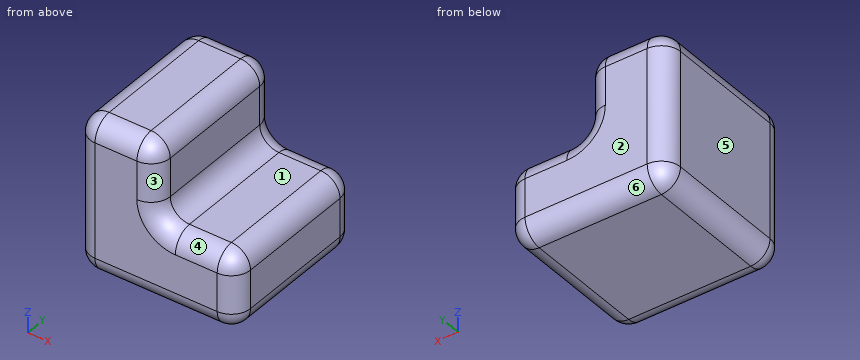
```python
from build123d import *

# Parameters (mm, degrees)
F0_W     = 83.6216490716
F0_H     = 83.1985995173
F1_DEPTH = 40
F2_W     = 41.8108245358
F2_H     = 83.1985995173
F3_DEPTH = 40
F4_F1_R  = 10
F4_F2_R  = 10


with BuildPart() as f1:
    # F0 (on Top) → F1 (new body)
    with BuildSketch(Plane.XY):
        with Locations((-17.3164242879, -4.335001111)):
            Rectangle(F0_W, F0_H)
    extrude(amount=F1_DEPTH)

    # F2 (on face) → F3 (join)
    with BuildSketch(Plane.XY.offset(40)):
        with Locations((-38.2218365557, -4.335001111)):
            Rectangle(F2_W, F2_H)
    extrude(amount=F3_DEPTH)

    # F4: fillet of radius 10 on 16 edges, made by hand

    # F4_f1
    f4_f1_edges = [f1.edges().sort_by_distance(p)[0] for p in [
        (-17.3164242879, -4.335001111, 40),
    ]]
    fillet(f4_f1_edges, radius=F4_F1_R)

    # F4_f2
    f4_f2_edges = [f1.edges().sort_by_distance(p)[0] for p in [
        (-17.3164242879, -4.335001111, 80),
        (-38.2218365557, -45.9343008697, 80),
        (-17.3164242879, -45.9343008697, 65),
        (-59.1272488236, -4.335001111, 80),
        (-38.2218365557, 37.2642986476, 80),
        (8.58898798, 37.2642986476, 40),
        (24.4944002479, -4.335001111, 40),
        (24.4944002479, -45.9343008697, 20),
        (24.4944002479, 37.2642986476, 20),
        (-17.3164242879, -45.9343008697, 0),
        (-59.1272488236, -45.9343008697, 40),
        (-59.1272488236, 37.2642986476, 40),
        (-59.1272488236, -4.335001111, 0),
        (-17.3164242879, 37.2642986476, 0),
        (24.4944002479, -4.335001111, 0),
        (-14.3874920997, 37.2642986476, 42.9289321881),
        (-14.3874920997, -45.9343008697, 42.9289321881),
    ]]
    fillet(f4_f2_edges, radius=F4_F2_R)


solid = f1.part
```
CAD build for the part. Positions are in the model's coordinates, mm. Face numbers are marked on the shaded views. A direction names the side the tool comes from. Round coordinates to 2 decimals unless told otherwise and drop trailing zeros. Loops run counter-clockwise (first coordinate to the right, second up) from the corner with the lowest first, then second, coordinate; pieces in that order, holes last. Notation, with made-up numbers: (9.5, 81.5) - (54.5, 81.5) arc R18 ccw to (54.5, 103.5) - close; hole circle Ø1 at (-23, 21). An arc over 180 degrees is marked (long way). Return JSON: item names as keys, results as strings. Group by question number.
Q1. Flat gauge pins, fed straight in: pin 1 Ø22 at (y, z) = (9.5, 58) entering from +X; pin 2 Ø11 at (x, y) = (2, 10.5) entering from +Z. Where does each tip first touch, or does it go through?
Q2. Two-plate mould, pull along Z, no slides. Class the marked faces 4, 5 and 6: +Z half, -Z half, draft (parallel to the pull), parting line (faces both ways), or undercut.
Q3. Band-saw the part on B-B on x = -1.5. Give the cut face in (y, z), plus the area to 3 significant figures.
Q4. Tool access for the marked faces 1, 2 and 3: list every direction of +Z, -Z, +X, -X, +Y, -Y with a clear straight run to the whole face (end or side of a thin tool).
Q5. Drill centre lines: line 1 along Z through (x, y) = (5.5, 0); line 2 along X through (y, z) = (24, 61); line 3 along Z through (x, y) = (-18.5, 3.5). Where is each one in solid material? Low to high. Write a range as [from, to].
Q6. Band-saw the part on A-A on z = 55. Give the cut face in (x, y), plus the area to 3 significant figures.
Q7. Band-saw the part on C-C on y = 0. Give the cut face in (x, z).
Solutions:
{
 "1": {"pin 1": "stops at x = -16.86", "pin 2": "stops at z = 40"},
 "2": {"face 4": "+Z half", "face 5": "draft", "face 6": "-Z half"},
 "3": {"outline": "(-45.93, 10) arc R10 ccw to (-35.93, 0) - (27.26, 0) arc R10 ccw to (37.26, 10) - (37.26, 30) arc R10 ccw to (27.26, 40) - (-35.93, 40) arc R10 ccw to (-45.93, 30) - close", "area": "3,240 mm^2"},
 "4": {"face 1": "+Z, +X, +Y, -Y", "face 2": "+Z, -Z, +X, -X, +Y", "face 3": "+Z, +X, -Y"},
 "5": {"line 1": "z = [0, 40]", "line 2": "x = [-59.13, -17.32]", "line 3": "z = [0, 74.72]"},
 "6": {"outline": "(-59.13, -35.93) arc R10 ccw to (-49.13, -45.93) - (-27.32, -45.93) arc R10 ccw to (-17.32, -35.93) - (-17.32, 27.26) arc R10 ccw to (-27.32, 37.26) - (-49.13, 37.26) arc R10 ccw to (-59.13, 27.26) - close", "area": "3,390 mm^2"},
 "7": {"outline": "(-59.13, 10) arc R10 ccw to (-49.13, 0) - (14.49, 0) arc R10 ccw to (24.49, 10) - (24.49, 30) arc R10 ccw to (14.49, 40) - (-7.32, 40) arc R10 cw to (-17.32, 50) - (-17.32, 70) arc R10 ccw to (-27.32, 80) - (-49.13, 80) arc R10 ccw to (-59.13, 70) - close"}
}
